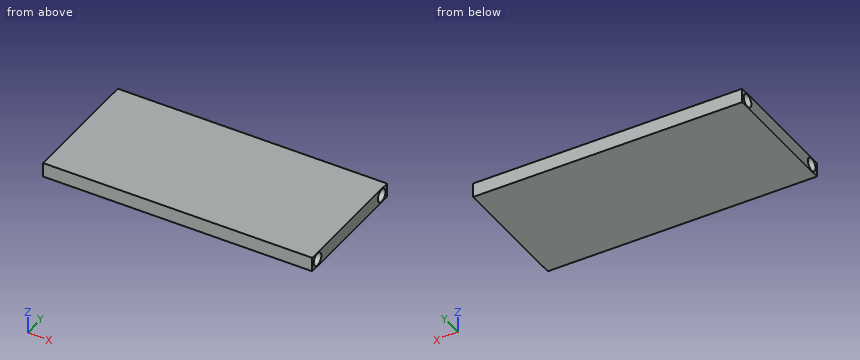
from build123d import *

# Parameters (mm, degrees)
BOSS_EXTRUDE1_DEPTH      = 4.064
BOSS_EXTRUDE1_DEPTH_BACK = 4.064
BOARD_W                  = 152.4
BOARD_H                  = 71.12
SKETCH2_R                = 3.6195
CUT_EXTRUDE1_DEPTH       = 157.546445811


with BuildPart() as part:
    # board → Boss-Extrude1 (new, two sides: drawn at the far end of the back side and taken through both)
    with BuildSketch(Plane.XY.offset(-BOSS_EXTRUDE1_DEPTH_BACK)):
        Rectangle(BOARD_W, BOARD_H)
    extrude(amount=BOSS_EXTRUDE1_DEPTH + BOSS_EXTRUDE1_DEPTH_BACK)

    # Sketch2 → Cut-Extrude1 (cut, through all)
    with BuildSketch(Plane(origin=(76.2, 0, 0), x_dir=(0, 0, -1), z_dir=(1, 0, 0))):
        with Locations((0, 30.48)):
            Circle(SKETCH2_R)
        with Locations((0, -30.48)):
            Circle(SKETCH2_R)
    extrude(amount=-CUT_EXTRUDE1_DEPTH, mode=Mode.SUBTRACT)


solid = part.part
Check sheet for the modelled part. Datum: model origin and axes. Units: mm. Round coordinates to 2 decimals unless told otherwise and drop trailing zeros. Write each loop counter-clockwise with the first axis right and the second up, starting at its lowest first coordinate (ties: lowest second). Pieces come first, ordered by that corner, then holes. Notation, with made-up numbers: (-5, 20.5) - (21, 20.5) arc R9 ccw to (21, 32.5) - close; hole circle Ø4 at (-9, 65). An arc over 180 degrees is marked (long way). Return JSON: item names as keys, results as strings.
Q1. Cross-section at C-C (x = -14.5). Record the boundary of the cut face in (y, z), then the cut area to 3 significant figures.
Returned:
{"outline": "(-35.56, -4.06) - (35.56, -4.06) - (35.56, 4.06) - (-35.56, 4.06) - close; hole circle Ø7.24 at (-30.48, 0); hole circle Ø7.24 at (30.48, 0)", "area": "496 mm²"}
Q2. Cross-section at B-B (z = 0). Record the boundary of the cut face in (x, y), then the cut area to 3 significant figures.
Returned:
{"outline": "(-76.2, -35.56) - (76.2, -35.56) - (76.2, -34.1) - (-76.2, -34.1) - close; (-76.2, -26.86) - (76.2, -26.86) - (76.2, 26.86) - (-76.2, 26.86) - close; (-76.2, 34.1) - (76.2, 34.1) - (76.2, 35.56) - (-76.2, 35.56) - close", "area": "8,630 mm²"}
Q3. Scan lines: L1, parallel to Y at x = 9.5, z = 0; L2, parallel to Y at x = -36.5, z = -1.5; L3, parallel to Z at x = 30, y = -30. Record each from-to range of solid material in increasing order. Write a range as from..to.
Returned:
{"L1": "y = -35.56..-34.1, -26.86..26.86, 34.1..35.56", "L2": "y = -35.56..-33.77, -27.19..27.19, 33.77..35.56", "L3": "z = -4.06..-3.59, 3.59..4.06"}
Q4. Cross-section at A-A (y = 30.48). Record the boundary of the cut face in (x, z).
Returned:
{"outline": "(-76.2, -4.06) - (76.2, -4.06) - (76.2, -3.62) - (-76.2, -3.62) - close; (-76.2, 3.62) - (76.2, 3.62) - (76.2, 4.06) - (-76.2, 4.06) - close"}
